Could you check a few things on this model? Use its own coordinates, in mm. A direction names the side the tool comes from. Round coordinates to 2 decimals unless told otherwise and drop trailing zeros. Loops run counter-clockwise (first coordinate to the right, second up) from the corner with the lowest first, then second, coordinate; pieces in that order, holes last. Notation, with made-up numbers: (52, 59.25) - (74, 59.25) arc R31 cw to (74, 94.25) - close; hole circle Ø7 at (51, 70.25). An arc over 180 degrees is marked (long way). Answer as CSV lines item,"result". Start each with the question number.
1) Suppose I cut it at C-C, the plane z = -30.5. Write out the boundary of the cut face in (x, y), then the cut area to 3 significant figures.
2) Please list where these lines run through material, in increasing order: line 1 along Z through (x, y) = (39.5, 32.05); line 2 along Z through (x, y) = (39.5, 33.8); line 3 along Z through (x, y) = (39.5, 27.75).
3) Which directions (+Z, -Z, +X, -X, +Y, -Y) give clear straight access to the entire face, cutting with the end or side of a thin tool? Please do faces 4 (the face through (-19.335, 33.535, -26.754)), 5 (the face through (32.5, 26, 11)), 6 (the face through (37, 26, -5.5)).
4) I'm going to push flat-ended pins straight in: pin 1 Ø5 at (x, y) = (39.5, 23.5) entering from -Z; pin 2 Ø4 at (x, z) = (12, 1.5) entering from -Y; pin 3 Ø8 at (x, y) = (-20, 28.5) entering from +Z. Where does each tip first touch, or does it pass through?
5) Suppose I cut it at B-B, the plane y = 32. Write out the boundary of the cut face in (x, z), then the cut area to 3 significant figures.
6) We'd pull the mould along X, two halves only. Please class faces 1 (the face through (-20, 26, -23.5)), 2 (the face through (37.7, 31, 12.2)), 3 (the face through (-43, 35, 34)): pulls with the +X half, pulls with the -X half, needs draft (parallel to the pull), parting line crosses it, or undercut.
7) Suppose I cut it at D-D, the plane z = -10.5. Write out the boundary of the cut face in (x, y), then the cut area to 3 significant figures.
8) Suppose I cut it at A-A, the plane x = 39.5. Write out the boundary of the cut face in (y, z), then the cut area to 3 significant figures.
```python
from build123d import *

# Parameters (mm, degrees)
SKETCH1_W           = 85
SKETCH1_H           = 67
BOSS_EXTRUDE1_DEPTH = 3
SKETCH1_3_W         = 89
SKETCH1_3_H         = 71
SKETCH1_3_W_2       = 85
SKETCH1_3_H_2       = 67
BOSS_EXTRUDE2_DEPTH = 50
CHAMFER1_SIZE       = 3
SKETCH2_W           = 10
SKETCH2_H           = 10
SKETCH2_R           = 2.1
BOSS_EXTRUDE3_DEPTH = 32
CUT_EXTRUDE1_START  = 3
SKETCH1_4_W         = 89
SKETCH1_4_H         = 71
SKETCH1_4_W_2       = 85
SKETCH1_4_H_2       = 67
CUT_EXTRUDE1_DEPTH  = 73.766087401
CUT_EXTRUDE2_START  = 15
SKETCH2_2_W         = 10
SKETCH2_2_H         = 10
SKETCH2_2_R         = 2.1
CUT_EXTRUDE2_DEPTH  = 51.303139281
SKETCH3_R           = 3.75
CUT_EXTRUDE3_DEPTH  = 5
CUT_EXTRUDE4_START  = 15
SKETCH4_W           = 102.54435907
SKETCH4_H           = 82.358611279
CUT_EXTRUDE4_DEPTH  = 40


with BuildPart() as part:
    # Sketch1 → Boss-Extrude1 (new body)
    with BuildSketch(Plane(origin=(0, 0, 0), x_dir=(1, 0, 0), z_dir=(0, 1, 0))):
        Rectangle(SKETCH1_W, SKETCH1_H)
    extrude(amount=BOSS_EXTRUDE1_DEPTH)

    # Sketch1<3> → Boss-Extrude2 (add)
    with BuildSketch(Plane(origin=(0, 0, 0), x_dir=(1, 0, 0), z_dir=(0, 1, 0))):
        Rectangle(SKETCH1_3_W, SKETCH1_3_H)
        Rectangle(SKETCH1_3_W_2, SKETCH1_3_H_2, mode=Mode.SUBTRACT)
    extrude(amount=BOSS_EXTRUDE2_DEPTH)

    # Chamfer1
    chamfer1_edges = [part.edges().sort_by_distance(p)[0] for p in [
        (-44.5, 25, -35.5),
        (-44.5, 25, 35.5),
        (44.5, 25, 35.5),
        (44.5, 25, -35.5),
    ]]
    chamfer(chamfer1_edges, length=CHAMFER1_SIZE)

    # Sketch2 → Boss-Extrude3 (add)
    # profile 1 of 3: a face of its own
    with BuildSketch(Plane(origin=(0, 3, 0), x_dir=(1, 0, 0), z_dir=(0, 1, 0))):
        with Locations((-19.5, 28.5)):
            Rectangle(SKETCH2_W, SKETCH2_H)
        with Locations(Location((-19.5, 30.5, 0), (0, 0, 90))):
            Circle(SKETCH2_R, mode=Mode.SUBTRACT)
    # profile 2 of 3: a face of its own
    with BuildSketch(Plane(origin=(0, 3, 0), x_dir=(1, 0, 0), z_dir=(0, 1, 0))):
        with Locations((37.5, 10.5)):
            Rectangle(SKETCH2_W, SKETCH2_H)
        with Locations(Location((39.5, 10.5, 0), (0, 0, 90))):
            Circle(SKETCH2_R, mode=Mode.SUBTRACT)
    # profile 3 of 3: a face of its own
    with BuildSketch(Plane(origin=(0, 3, 0), x_dir=(1, 0, 0), z_dir=(0, 1, 0))):
        with Locations((37.5, -10.5)):
            Rectangle(SKETCH2_W, SKETCH2_H)
        with Locations(Location((39.5, -10.5, 0), (0, 0, 90))):
            Circle(SKETCH2_R, mode=Mode.SUBTRACT)
    extrude(amount=BOSS_EXTRUDE3_DEPTH)

    # Sketch1<4> → Cut-Extrude1 (cut, through all)
    with BuildSketch(Plane(origin=(0, 0, 0), x_dir=(1, 0, 0), z_dir=(0, 1, 0)).offset(CUT_EXTRUDE1_START)):
        Rectangle(SKETCH1_4_W, SKETCH1_4_H)
        Rectangle(SKETCH1_4_W_2, SKETCH1_4_H_2, mode=Mode.SUBTRACT)
    extrude(amount=CUT_EXTRUDE1_DEPTH, mode=Mode.SUBTRACT)

    # Sketch2<2> → Cut-Extrude2 (cut, through all)
    # profile 1 of 3: a face of its own
    with BuildSketch(Plane(origin=(0, 3, 0), x_dir=(1, 0, 0), z_dir=(0, 1, 0)).offset(CUT_EXTRUDE2_START)):
        with Locations((-19.5, 28.5)):
            Rectangle(SKETCH2_2_W, SKETCH2_2_H)
        with Locations(Location((-19.5, 30.5, 0), (0, 0, 90))):
            Circle(SKETCH2_2_R, mode=Mode.SUBTRACT)
    # profile 2 of 3: a face of its own
    with BuildSketch(Plane(origin=(0, 3, 0), x_dir=(1, 0, 0), z_dir=(0, 1, 0)).offset(CUT_EXTRUDE2_START)):
        with Locations((37.5, 10.5)):
            Rectangle(SKETCH2_2_W, SKETCH2_2_H)
        with Locations(Location((39.5, 10.5, 0), (0, 0, 90))):
            Circle(SKETCH2_2_R, mode=Mode.SUBTRACT)
    # profile 3 of 3: a face of its own
    with BuildSketch(Plane(origin=(0, 3, 0), x_dir=(1, 0, 0), z_dir=(0, 1, 0)).offset(CUT_EXTRUDE2_START)):
        with Locations((37.5, -10.5)):
            Rectangle(SKETCH2_2_W, SKETCH2_2_H)
        with Locations(Location((39.5, -10.5, 0), (0, 0, 90))):
            Circle(SKETCH2_2_R, mode=Mode.SUBTRACT)
    extrude(amount=CUT_EXTRUDE2_DEPTH, mode=Mode.SUBTRACT)

    # Sketch3 → Cut-Extrude3 (cut)
    with BuildSketch(Plane.XZ):
        with Locations(Location((-19.5, -30.5, 0), (0, 0, 270))):
            Circle(SKETCH3_R)
        with Locations(Location((39.5, -10.5, 0), (0, 0, 270))):
            Circle(SKETCH3_R)
        with Locations(Location((39.5, 10.5, 0), (0, 0, 270))):
            Circle(SKETCH3_R)
    extrude(amount=-CUT_EXTRUDE3_DEPTH, mode=Mode.SUBTRACT)

    # Mirror5: part across plane


with BuildPart() as part_1:
    add(part.part)
    add(part.part.mirror(Plane.ZX.offset(18)))

    # Sketch4 → Cut-Extrude4 (cut)
    with BuildSketch(Plane.XZ.offset(-33).offset(CUT_EXTRUDE4_START)):
        with Locations((-1.663138354, 2.062291559)):
            Rectangle(SKETCH4_W, SKETCH4_H)
    extrude(amount=CUT_EXTRUDE4_DEPTH, mode=Mode.SUBTRACT)


solid = part_1.part
```
Filled sheet:
1,outline,"(-44.5, 33) - (-24.5, 33) - (-24.5, 18) - (-21.6, 18) - (-21.6, 31) - (-23.25, 31) - (-23.25, 36) - (-44.5, 36) - close; (-17.4, 18) - (-14.5, 18) - (-14.5, 33) - (44.5, 33) - (44.5, 36) - (-15.75, 36) - (-15.75, 31) - (-17.4, 31) - close"
1,area,"325 mm²"
2,line 1,"-15.5 to -14.25, -6.75 to -5.5, 5.5 to 6.75, 14.25 to 15.5"
2,line 2,"-35.5 to -14.25, -6.75 to 6.75, 14.25 to 35.5"
2,line 3,"-15.5 to -12.6, -8.4 to -5.5, 5.5 to 8.4, 12.6 to 15.5"
3,face 4,"+Y"
3,face 5,"+Z, -Z, -X, -Y"
3,face 6,"+X, -X, -Y"
4,pin 1,"z = -15.5"
4,pin 2,"y = 33"
4,pin 3,"z = -23.5"
5,outline,"(-24.5, -33.5) - (-21.75, -33.5) arc R3.75 cw (long way) to (-17.25, -33.5) - (-14.5, -33.5) - (-14.5, -23.5) - (-24.5, -23.5) - close; (32.5, -15.5) - (42.5, -15.5) - (42.5, -12.75) arc R3.75 cw (long way) to (42.5, -8.25) - (42.5, -5.5) - (32.5, -5.5) - close; (32.5, 5.5) - (42.5, 5.5) - (42.5, 8.25) arc R3.75 cw (long way) to (42.5, 12.75) - (42.5, 15.5) - (32.5, 15.5) - close"
5,area,"174 mm²"
6,face 1,"needs draft"
6,face 2,"undercut"
6,face 3,"pulls with the -X half"
7,outline,"(-44.5, 33) - (32.5, 33) - (32.5, 18) - (37.4, 18) - (37.4, 31) - (35.75, 31) - (35.75, 36) - (-44.5, 36) - close; (41.6, 18) - (42.5, 18) - (42.5, 31) - (41.6, 31) - close; (43.25, 33) - (44.5, 33) - (44.5, 36) - (43.25, 36) - close"
7,area,"326 mm²"
8,outline,"(18, -15.5) - (33, -15.5) - (33, -35.5) - (36, -35.5) - (36, -14.25) - (31, -14.25) - (31, -12.6) - (18, -12.6) - close; (18, -8.4) - (31, -8.4) - (31, -6.75) - (36, -6.75) - (36, 6.75) - (31, 6.75) - (31, 8.4) - (18, 8.4) - (18, 5.5) - (33, 5.5) - (33, -5.5) - (18, -5.5) - close; (18, 12.6) - (31, 12.6) - (31, 14.25) - (36, 14.25) - (36, 35.5) - (33, 35.5) - (33, 15.5) - (18, 15.5) - close"
8,area,"329 mm²"
